```python
from build123d import *

# Parameters (mm, degrees)
SKETCH1_W             = 74
SKETCH1_H             = 57.1
BOSS_EXTRUDE1_DEPTH   = 80
FILLET1_R             = 2
CUT_EXTRUDE1_REACH    = 94.65
SKETCH2_R             = 5.23
SKETCH7_W             = 20
SKETCH7_H             = 57.1
BOSS_EXTRUDE2_DEPTH   = 15
M8_TAPPED_HOLE1_D     = 6.8
FILLET2_R             = 5
F_8_0MM_DOWEL_HOLE1_D = 8


# Read off the part's stored shape, not the designer's step: Draft1
with BuildPart() as part:
    # Sketch1 → Boss-Extrude1 (new body)
    with BuildSketch(Plane(origin=(0, 0, 0), x_dir=(1, 0, 0), z_dir=(0, 1, 0))):
        Rectangle(SKETCH1_W, SKETCH1_H)
    extrude(amount=BOSS_EXTRUDE1_DEPTH)

    # Fillet1
    fillet1_edges = [part.edges().sort_by_distance(p)[0] for p in [
        (-37, 80, 0),
        (37, 80, 0),
    ]]
    fillet(fillet1_edges, radius=FILLET1_R)

    # Sketch2 → Cut-Extrude1 (cut, up to next)
    with BuildSketch(Plane(origin=(0, 80, 0), x_dir=(1, 0, 0), z_dir=(0, 1, 0)), mode=Mode.PRIVATE) as cut_extrude1_sk1:
        with Locations(Location((0, 0, 0), (0, 0, 270))):
            Circle(SKETCH2_R)
    cut_extrude1_tool1 = extrude(cut_extrude1_sk1.sketch, amount=-CUT_EXTRUDE1_REACH, mode=Mode.PRIVATE) & part.part
    add(cut_extrude1_tool1.solids().sort_by_distance((0, 80, 0))[0], mode=Mode.SUBTRACT)

    # Draft1 outline → Draft1 (revolve, cut)
    with BuildSketch(Plane.XY):
        Polygon((6.570548986, 0), (5.23, 76.8), (5.23, 0), align=None)
    revolve(axis=Axis((0, 0, 0), (0, 1, 0)), mode=Mode.SUBTRACT)

    # Sketch7 → Boss-Extrude2 (add)
    with BuildSketch(Plane.XZ):
        with Locations((-47, 0)):
            Rectangle(SKETCH7_W, SKETCH7_H)
    boss_extrude2 = extrude(amount=-BOSS_EXTRUDE2_DEPTH)

    # Mirror1: Boss-Extrude2 across plane
    add(boss_extrude2.mirror(Plane(origin=(0, 0, 0), x_dir=(0, 0, 1), z_dir=(1, 0, 0))))

    # M8 Tapped Hole1 (through all)
    with Locations(Plane(origin=(0, 0, 0), x_dir=(-1, 0, 0), z_dir=(0, -1, 0))):
        with Locations((-49, 20.55), (49, 20.55), (49, -20.55), (-49, -20.55)):
            Hole(M8_TAPPED_HOLE1_D / 2)

    # Fillet2
    fillet2_edges = [part.edges().sort_by_distance(p)[0] for p in [
        (-37, 15, 0),
        (37, 15, 0),
    ]]
    fillet(fillet2_edges, radius=FILLET2_R)

    # Ø8.0mm Dowel Hole1 (through all)
    with Locations(Plane(origin=(0, 0, 0), x_dir=(-1, 0, 0), z_dir=(0, -1, 0))):
        with Locations((-49, 0), (49, 0)):
            Hole(F_8_0MM_DOWEL_HOLE1_D / 2)


solid = part.part
```
Check sheet for the modelled part. Datum: model origin and axes. Units: mm. A direction names the side the tool comes from. Coordinates: 2 decimals unless noted, no trailing zeros. Order: outer loops, then holes, each group sorted by start corner. A loop starts at its lowest first (then second) coordinate and runs counter-clockwise, first axis right, second up. Notation, with made-up numbers: M 0,84.25 L 59,84.25 A15 cw 59,90.25 Z; hole C -13.75,23 d7. An arc over 180 degrees is marked long. Write each question's results on one line, items separated by ' | '. Start each with the question number.
1. Cross-section at A-A on x = -49. Record the cut outline in (y, z).
2. Cross-section at B-B on z = 20.55. Record the cut outline in (x, y), and give its area (4 significant figures).
3. Cross-section at C-C on y = 73. Record the cut outline in (x, z), and give its area (3 significant figures).
4. Cross-section at D-D on z = 0. State how many separate pieces and enclosed holes the cut face has, and give its area (3 significant figures).
5. Material ranges on probe 1 along Z at (x, y) = (49, 8.25); probe 2 along X at (y, z) = (10.5, 20.55); probe 3 along X at (y, z) = (38.5, -10), recorded low to high.
6. Go/stop test with flat-tipped pins: P1, Ø2, axis at y = 56.5, z = 12, coming from the +X side; P2, Ø12, axis at x = 47.5, z = -12, coming from the +Y side; P3, Ø4, axis at x = -41, z = 8, coming from the +Y side. Record where each tip stops, or that it passes through.
7. Mould release check, pull along X, two halves, no side actions. Record for faces 1 (the face through (1, 0, 7)), 2 (the face through (39, 16, 0)), 3 (the face through (-45.86, 7.6, 21.85)): +X half, -X half, draft (parallel to the pull), parting line (faces both ways), or undercut.
8. Access from +Z, -Z, +X, -X, +Y, -Y to the whole of each face (thin tool, end or side, straight path). Record for faces 4 (the face through (-55, 15, 0)), 5 (the face through (2.718, 38.938, 5.226)), 6 (the face through (37, 49, 0)).
Checks:
1) outline: M 0,-28.55 L 15,-28.55 L 15,-23.95 L 0,-23.95 Z; M 0,-17.15 L 15,-17.15 L 15,-4 L 0,-4 Z; M 0,4 L 15,4 L 15,17.15 L 0,17.15 Z; M 0,23.95 L 15,23.95 L 15,28.55 L 0,28.55 Z
2) outline: M -57,0 L -52.4,0 L -52.4,15 L -57,15 Z; M -45.6,0 L 45.6,0 L 45.6,15 L 42,15 A5 cw 37,20 L 37,78 A2 ccw 35,80 L -35,80 A2 ccw -37,78 L -37,20 A5 cw -42,15 L -45.6,15 Z; M 52.4,0 L 57,0 L 57,15 L 52.4,15 Z | area: 6,325 mm²
3) outline: M -37,-28.55 L 37,-28.55 L 37,28.55 L -37,28.55 Z; hole C 0,0 d10.59 | area: 4,140 mm²
4) separate pieces: 4 | enclosed holes: 0 | area: 5,350 mm²
5) probe 1: z = -28.55 to -23.95, -17.15 to -4, 4 to 17.15, 23.95 to 28.55 | probe 2: x = -57 to -52.4, -45.6 to 45.6, 52.4 to 57 | probe 3: x = -37 to 37
6) P1: stops at x = 37 | P2: stops at y = 15.03 | P3: stops at y = 16
7) face 1: draft | face 2: +X half | face 3: undercut
8) face 4: +Z, -Z, -X, +Y | face 5: -Y | face 6: +Z, -Z, +X, +Y
